The figure shows three views and two pictorial views of one solid part (mm, origin at its lowest corner). Answer the questions. A direction names the side the tool comes from. Give positions to 0.01 mm unless a question says otherwise; leave off trailing zeros. Loops run counter-clockwise (first coordinate to the right, second up) from the corner with the lowest first, then second, coordinate; pieces in that order, holes last. Notation, with made-up numbers: (-20.75, 42) -> (31.25, 42) arc R24 ccw to (31.25, 81) -> close; hole circle Ø11 at (33.5, 89.25). An arc over 180 degrees is marked (long way). Answer as CSV lines item,"result". Start each with the question number.
1. Find section D-D, the plane x = 57.5. Give the vertices of the cut face in (y, z), and give its area (3 significant figures).
2. Find section C-C, the plane z = 5. Count the separate pieces of the cut face and the enclosed holes in it.
3. Find section A-A, the plane y = 13.5. Give the vertices of the cut face in (x, z), and give its area (3 significant figures).
4. Find section B-B, the plane x = 28.5. Give the vertices of the cut face in (y, z), and give its area (3 significant figures).
5. A tool of negligible diameter and unlimited length cuts with its end or side. For the marked faces 1 and 2, from which of +Z, -Z, +X, -X, +Y, -Y can it reach the whole face along a straight path? Write none if from no direction.
6. Flat-ended cylindrical pins translate along their axes: pin 1 Ø1.9 at (x, z) = (65, 2.5) entering from +Y; pin 2 Ø3 at (y, z) = (74, 3) entering from +X. Find the tip coordinate at first contact, or state that the pin passes through.
7. Find the intervals of material crossed by line 1 along X through (y, z) = (28, 4); line 2 along X through (y, z) = (12, 5); line 3 along X through (y, z) = (89, 4.75) (1 decimal), in increasing order.
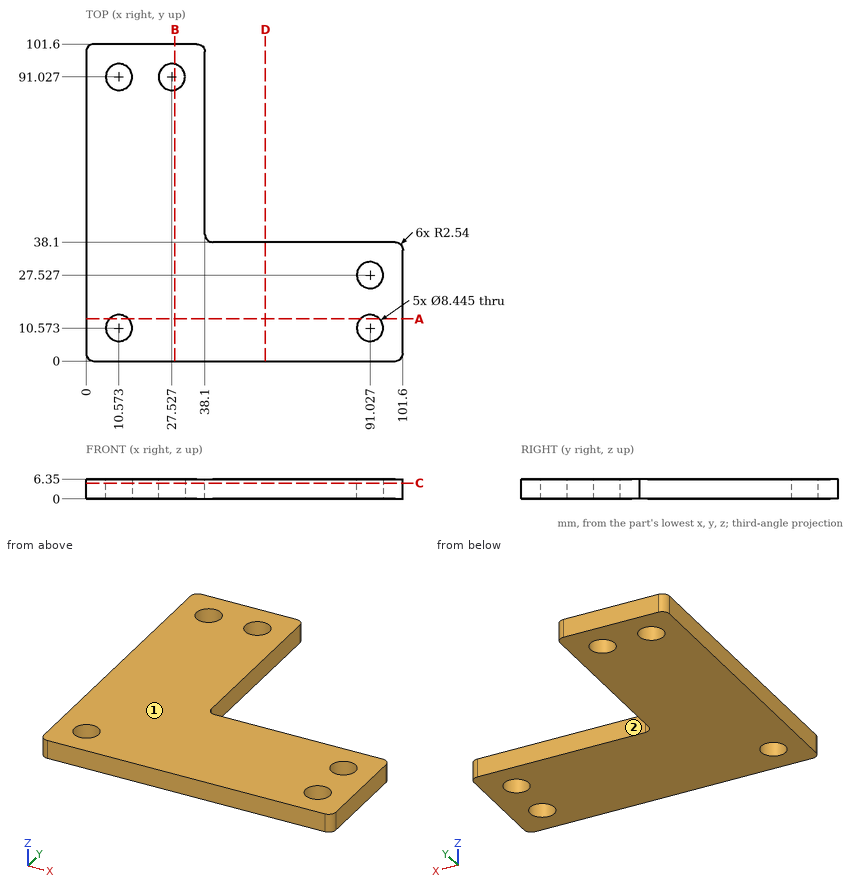
Resolved:
1,outline,"(0, 0) -> (38.1, 0) -> (38.1, 6.35) -> (0, 6.35) -> close"
1,area,"242 mm^2"
2,separate pieces,"1"
2,enclosed holes,"5"
3,outline,"(0, 0) -> (7.53, 0) -> (7.53, 6.35) -> (0, 6.35) -> close; (13.62, 0) -> (87.98, 0) -> (87.98, 6.35) -> (13.62, 6.35) -> close; (94.07, 0) -> (101.6, 0) -> (101.6, 6.35) -> (94.07, 6.35) -> close"
3,area,"568 mm^2"
4,outline,"(0, 0) -> (86.92, 0) -> (86.92, 6.35) -> (0, 6.35) -> close; (95.14, 0) -> (101.6, 0) -> (101.6, 6.35) -> (95.14, 6.35) -> close"
4,area,"593 mm^2"
5,face 1,"+Z, +X, -X, +Y, -Y"
5,face 2,"+Z, -Z, +X, +Y"
6,pin 1,"stops at y = 38.1"
6,pin 2,"stops at x = 38.1"
7,line 1,"x = 0 to 86.83, 95.22 to 101.6"
7,line 2,"x = 0 to 6.6, 14.55 to 87.05, 95 to 101.6"
7,line 3,"x = 0 to 6.9, 14.3 to 23.8, 31.2 to 38.1"
